Could you check a few things on this model? Use its own coordinates, in mm. A direction names the side the tool comes from. Give positions to 0.01 mm unless a question says otherwise; leave off trailing zeros. Loops run counter-clockwise (first coordinate to the right, second up) from the corner with the lowest first, then second, coordinate; pieces in that order, holes last. Notation, with made-up numbers: M 34,34.5 L 77,34.5 A21 cw 77,60.5 Z; hole C -34,-2.75 d1. An arc over 180 degrees is marked long. Answer in a Markdown table with one row per item. Add a question column.
```python
from build123d import *

# Parameters (mm, degrees)
F0_R     = 1.49987
F0_R_2   = 11
F0_W     = 6.35
F0_H     = 6.35
F1_DEPTH = 6.35
F2_R     = 1.27


with BuildPart() as f1:
    # F0 (on Top) → F1 (new body)
    with BuildSketch(Plane.XY):
        Polygon((23.876, 22.225), (-23.876, 22.225), (-23.876, 12.7), (-23.876, 6.35), (-23.876, -6.35), (-23.876, -12.7), (-23.876, -22.225), (23.876, -22.225), (23.876, -12.7), (23.876, -6.35), (23.876, 6.35), (23.876, 12.7), align=None)
        with Locations((-15.52, -15.52)):
            Circle(F0_R, mode=Mode.SUBTRACT)
        with Locations((15.52, -15.52)):
            Circle(F0_R, mode=Mode.SUBTRACT)
        with Locations((-15.52, 15.52)):
            Circle(F0_R, mode=Mode.SUBTRACT)
        Circle(F0_R_2, mode=Mode.SUBTRACT)
        with Locations((15.52, 15.52)):
            Circle(F0_R, mode=Mode.SUBTRACT)
        with Locations((-27.051, 9.525)):
            Rectangle(F0_W, F0_H)
        with Locations((27.051, 9.525)):
            Rectangle(F0_W, F0_H)
        with Locations((-27.051, -9.525)):
            Rectangle(F0_W, F0_H)
        with Locations((27.051, -9.525)):
            Rectangle(F0_W, F0_H)
    extrude(amount=F1_DEPTH)

    # F2
    f2_edges = [f1.edges().sort_by_distance(p)[0] for p in [
        (-23.876, -22.225, 3.175),
        (23.876, -22.225, 3.175),
        (23.876, 22.225, 3.175),
        (-23.876, 22.225, 3.175),
        (30.226, -12.7, 3.175),
        (30.226, -6.35, 3.175),
        (30.226, 6.35, 3.175),
        (30.226, 12.7, 3.175),
        (-30.226, 12.7, 3.175),
        (-30.226, 6.35, 3.175),
        (-30.226, -6.35, 3.175),
        (-30.226, -12.7, 3.175),
    ]]
    fillet(f2_edges, radius=F2_R)


solid = f1.part
```
Item 1: If we mould it in two halves opening along X, with no side actions, what happens to faces 1 (the face through (23.494, 21.863, 3.219)), 2 (the face through (14.41, 16.53, 3.13)), 3 (the face through (0, 22.225, 3))? For each: +X half, -X half, draft (parallel to the pull), parting line (faces both ways), or undercut.
Item 2: Suppose I cut it at A-A (x = -15.52). List the corners of the cut face in (y, z) for me (3 decimals), then the cut area to 3 significant figures.
Item 3: I need wall thicknesses on L1, parallel to Y at x = 15.52, z = 2.5 (3 decimals); L2, parallel to X at y = -16, z = 5.5; L3, parallel to Y at x = -27, z = 0.5. Which ranges of each line are inside material? Lowest first, please.
Item 4: Suppose I cut it at B-B (y = -15.52). List the corners of the cut face in (x, z) for me, then the cut area to 3 significant figures.
Item 5: Suppose I cut it at D-D (y = -1.5). List the corners of the cut face in (x, z) for me.
Item 6: Suppose I cut it at C-C (x = 0). List the corners of the cut face in (y, z) for me (3 decimals), then the cut area to 3 significant figures.
Item 7: For faces 4 (the face through (-29.86, 6.73, 3.22)), 5 (the face through (-26, -12.7, 3)), 6 (the face through (23.876, 0, 3)), which set-ups out of +Z, -Z, +X, -X, +Y, -Y let a thin tool reach every point of the face, with its end or its side?
Item 8: For P1, Ø1.9, axis at y = 15.5, z = 3, coming from the +X side; P2, Ø3, axis at y = -16.5, z = 2, coming from the -X side; P3, Ø2.5, axis at x = 15.52, y = 15.52, coming from the +Z side; P4, Ø1.5, axis at x = 27, z = 2, coming from the -Y side, each with a flat end and sliding along its axis, tell me the tip position at first contact or that it passes through.
Values found:
| question | item | result |
|---|---|---|
| 1 | face 1 | +X half |
| 1 | face 2 | undercut |
| 1 | face 3 | draft |
| 2 | outline | M -22.225,0 L -17.02,0 L -17.02,6.35 L -22.225,6.35 Z; M -14.02,0 L 14.02,0 L 14.02,6.35 L -14.02,6.35 Z; M 17.02,0 L 22.225,0 L 22.225,6.35 L 17.02,6.35 Z |
| 2 | area | 244 mm² |
| 3 | L1 | -22.225 to -17.02, -14.02 to 14.02, 17.02 to 22.225 |
| 3 | L2 | -23.88 to -16.94, -14.1 to 14.1, 16.94 to 23.88 |
| 3 | L3 | -12.7 to -6.35, 6.35 to 12.7 |
| 4 | outline | M -23.88,0 L -17.02,0 L -17.02,6.35 L -23.88,6.35 Z; M -14.02,0 L 14.02,0 L 14.02,6.35 L -14.02,6.35 Z; M 17.02,0 L 23.88,0 L 23.88,6.35 L 17.02,6.35 Z |
| 4 | area | 265 mm² |
| 5 | outline | M -23.88,0 L -10.9,0 L -10.9,6.35 L -23.88,6.35 Z; M 10.9,0 L 23.88,0 L 23.88,6.35 L 10.9,6.35 Z |
| 6 | outline | M -22.225,0 L -11,0 L -11,6.35 L -22.225,6.35 Z; M 11,0 L 22.225,0 L 22.225,6.35 L 11,6.35 Z |
| 6 | area | 143 mm² |
| 7 | face 4 | +Z, -Z, -X |
| 7 | face 5 | +Z, -Z, -X, -Y |
| 7 | face 6 | +Z, -Z, +X |
| 8 | P1 | x = 23.88 |
| 8 | P2 | x = -23.88 |
| 8 | P3 | through |
| 8 | P4 | y = -12.7 |
